Geometry check sheet. Reference: the model listing, model coordinates, mm. Face numbers are marked on the shaded views. A direction names the side the tool comes from. Round coordinates to 2 decimals unless told otherwise and drop trailing zeros. Order: outer loops, then holes, each group sorted by start corner. A loop starts at its lowest first (then second) coordinate and runs counter-clockwise, first axis right, second up.
```python
from build123d import *

# Parameters (mm, degrees)
BOSS_EXTRUDE1_DEPTH                 = 10
SKETCH3_R                           = 3.5
IZVRTINA_VIJACENJE_NOSILCA_M7_DEPTH = 10
BOSS_EXTRUDE2_DEPTH                 = 30
SKETCH8_W                           = 200
SKETCH8_H                           = 30
IZVRTINA_KABLI_DEPTH                = 5
SKETCH10_R                          = 1.5
IZVRTINE_RPI_M2_5_HEAT_INSERT_DEPTH = 10
SKETCH11_R                          = 1.5
IZVRTINE_BUCK_M2_HEAT_INSERTS_DEPTH = 10
SKETCH12_R                          = 1.5
IZVRTINE_UNO_M2_5_HEAT_INSERT_DEPTH = 10
SKETCH14_R                          = 2.5
IZVRTINE_TOP_M4_HEAT_INSERT_DEPTH   = 6


with BuildPart() as part:
    # Sketch2 → Boss-Extrude1 (new body)
    with BuildSketch(Plane.XY):
        with BuildLine():
            Line((52.5, 60), (-52.5, 60))
            Line((-52.5, 60), (-52.5, 68))
            ThreePointArc((-52.5, 68), (-60, 75.5), (-67.5, 68))
            Line((-67.5, 68), (-67.5, 60))
            Line((-67.5, 60), (-115, 60))
            ThreePointArc((-115, 60), (-118.535533906, 58.535533906), (-120, 55))
            Line((-120, 55), (-120, -55))
            ThreePointArc((-120, -55), (-118.535533906, -58.535533906), (-115, -60))
            Line((-115, -60), (-67.5, -60))
            Line((-67.5, -60), (-67.5, -68))
            ThreePointArc((-67.5, -68), (-60, -75.5), (-52.5, -68))
            Line((-52.5, -68), (-52.5, -60))
            Line((-52.5, -60), (52.5, -60))
            Line((52.5, -60), (52.5, -68))
            ThreePointArc((52.5, -68), (60, -75.5), (67.5, -68))
            Line((67.5, -68), (67.5, -60))
            Line((67.5, -60), (115, -60))
            ThreePointArc((115, -60), (118.535533906, -58.535533906), (120, -55))
            Line((120, -55), (120, 55))
            ThreePointArc((120, 55), (118.535533906, 58.535533906), (115, 60))
            Line((115, 60), (67.5, 60))
            Line((67.5, 60), (67.5, 68))
            ThreePointArc((67.5, 68), (60, 75.5), (52.5, 68))
            Line((52.5, 68), (52.5, 60))
        make_face()
    extrude(amount=BOSS_EXTRUDE1_DEPTH)

    # Sketch3 → izvrtina_vijacenje_nosilca_m7 (cut)
    with BuildSketch(Plane.XY.offset(10)):
        with Locations((-60, 68)):
            Circle(SKETCH3_R)
        with Locations((-60, -68)):
            Circle(SKETCH3_R)
        with Locations((60, -68)):
            Circle(SKETCH3_R)
        with Locations((60, 68)):
            Circle(SKETCH3_R)
    extrude(amount=-IZVRTINA_VIJACENJE_NOSILCA_M7_DEPTH, mode=Mode.SUBTRACT)

    # Sketch7 → Boss-Extrude2 (add)
    with BuildSketch(Plane.XY.offset(10)):
        with BuildLine():
            Line((-115, -60), (115, -60))
            ThreePointArc((115, -60), (118.535533906, -58.535533906), (120, -55))
            Line((120, -55), (120, 55))
            ThreePointArc((120, 55), (118.535533906, 58.535533906), (115, 60))
            Line((115, 60), (-115, 60))
            ThreePointArc((-115, 60), (-118.535533906, 58.535533906), (-120, 55))
            Line((-120, 55), (-120, -55))
            ThreePointArc((-120, -55), (-118.535533906, -58.535533906), (-115, -60))
        make_face()
        with BuildLine():
            Line((-112.5, 50), (-112.5, -50))
            ThreePointArc((-112.5, -50), (-111.035533906, -53.535533906), (-107.5, -55))
            Line((-107.5, -55), (107.5, -55))
            ThreePointArc((107.5, -55), (111.035533906, -53.535533906), (112.5, -50))
            Line((112.5, -50), (112.5, 50))
            ThreePointArc((112.5, 50), (111.035533906, 53.535533906), (107.5, 55))
            Line((107.5, 55), (-107.5, 55))
            ThreePointArc((-107.5, 55), (-111.035533906, 53.535533906), (-112.5, 50))
        make_face(mode=Mode.SUBTRACT)
    extrude(amount=BOSS_EXTRUDE2_DEPTH)

    # Sketch8 → izvrtina_kabli (cut)
    with BuildSketch(Plane.XZ.offset(60)):
        with Locations((0, 25)):
            Rectangle(SKETCH8_W, SKETCH8_H)
    extrude(amount=-IZVRTINA_KABLI_DEPTH, mode=Mode.SUBTRACT)

    # Sketch10 → izvrtine_rpi_m2.5_heat_insert (cut)
    with BuildSketch(Plane.XY.offset(10)):
        with Locations((24.5, 40.5)):
            Circle(SKETCH10_R)
        with Locations((24.5, -17.5)):
            Circle(SKETCH10_R)
        with Locations((-24.5, -17.5)):
            Circle(SKETCH10_R)
        with Locations((-24.5, 40.5)):
            Circle(SKETCH10_R)
    extrude(amount=-IZVRTINE_RPI_M2_5_HEAT_INSERT_DEPTH, mode=Mode.SUBTRACT)

    # Sketch11 → izvrtine_buck_m2_heat_inserts (cut)
    with BuildSketch(Plane.XY.offset(10)):
        with Locations((-87, 8)):
            Circle(SKETCH11_R)
        with Locations((-65, 8)):
            Circle(SKETCH11_R)
        with Locations((-65, -39)):
            Circle(SKETCH11_R)
        with Locations((-87, -39)):
            Circle(SKETCH11_R)
    extrude(amount=-IZVRTINE_BUCK_M2_HEAT_INSERTS_DEPTH, mode=Mode.SUBTRACT)

    # Sketch12 → izvrtine_uno_m2.5_heat_insert (cut)
    with BuildSketch(Plane.XY.offset(10)):
        with Locations((75, 34)):
            Circle(SKETCH12_R)
        with Locations((75, -8)):
            Circle(SKETCH12_R)
    extrude(amount=-IZVRTINE_UNO_M2_5_HEAT_INSERT_DEPTH, mode=Mode.SUBTRACT)

    # Sketch14 → izvrtine_top_m4_heat_insert (cut)
    with BuildSketch(Plane.XY.offset(40)):
        with Locations((-115, 55)):
            Circle(SKETCH14_R)
        with Locations((115, 55)):
            Circle(SKETCH14_R)
        with Locations((115, -55)):
            Circle(SKETCH14_R)
        with Locations((-115, -55)):
            Circle(SKETCH14_R)
    extrude(amount=-IZVRTINE_TOP_M4_HEAT_INSERT_DEPTH, mode=Mode.SUBTRACT)


solid = part.part
```
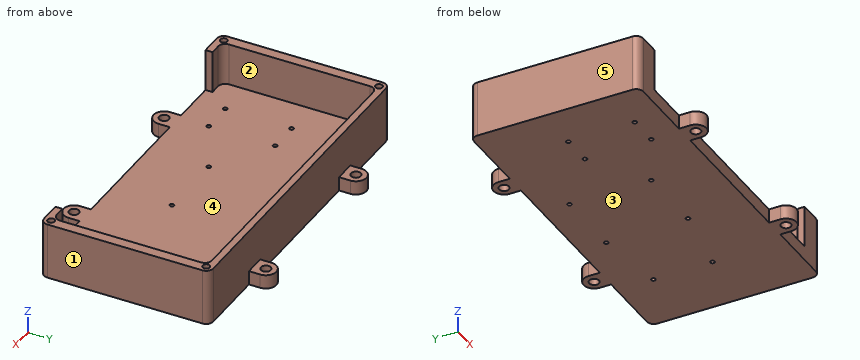
(1) Draft check along X on the marked faces 3, 4 and 5. Enter one of: released by +X, released by -X, zero draft, split by the parting line, or undercut.
Returned:
face 3: zero draft
face 4: undercut
face 5: released by -X
(2) Material ranges on line 1 (Y direction, x = -115, z = 38); line 2 (X direction, y = -22, z = 36.5); line 3 (Y direction, x = -24, z = 4), recorded low to high.
Returned:
line 1: y = -60 to -57.5, -52.5 to 52.5, 57.5 to 60
line 2: x = -120 to -112.5, 112.5 to 120
line 3: y = -60 to -18.91, -16.09 to 39.09, 41.91 to 60
(3) Depth check by flat-ended pin: P1, Ø4, axis at y = -57.5, z = 29, coming from the +X side; P2, Ø5, axis at x = -65, y = 8, coming from the +Z side; P3, Ø12, axis at x = 83.5, z = 7.5, coming from the -Y side; P4, Ø5.5, axis at x = -60, y = 68, coming from the -Z side. Enter the tip coordinate at first touch or a pass-through.
Returned:
P1: stops at x = 119.97
P2: stops at z = 10
P3: stops at y = -60
P4: passes through
(4) Set-up check for the marked faces 1 and 2: record each of +Z, -Z, +X, -X, +Y, -Y from which the full face is reachable in a straight line by a thin tool's end or side.
Returned:
face 1: +Z, -Z, +X, +Y, -Y
face 2: +Z
(5) Sectioned sample at C-C, the plane z = 3.5. Give the number of separate pieces and of enclosed holes in the cut face, and give its area (3 significant figures).
Returned:
separate pieces: 1
enclosed holes: 14
area: 29,400 mm2
(6) Sectioned sample at B-B, the plane x = -93.5. Record the cut outline in (y, z).
Returned:
outline: (-60, 0) - (60, 0) - (60, 40) - (55, 40) - (55, 10) - (-60, 10) - close
(7) Sectioned sample at A-A, the plane z = 21.5. Record the cut outline in (x, y).
Returned:
outline: (-120, -55) arc R5 ccw to (-115, -60) - (-100, -60) - (-100, -55) - (-107.5, -55) arc R5 cw to (-112.5, -50) - (-112.5, 50) arc R5 cw to (-107.5, 55) - (107.5, 55) arc R5 cw to (112.5, 50) - (112.5, -50) arc R5 cw to (107.5, -55) - (100, -55) - (100, -60) - (115, -60) arc R5 ccw to (120, -55) - (120, 55) arc R5 ccw to (115, 60) - (-115, 60) arc R5 ccw to (-120, 55) - close
